```python
from build123d import *

# Parameters (mm, degrees)
BOSS_EXTRUDE1_DEPTH       = 38
BOSS_EXTRUDE1_2_DEPTH     = 38
SKETCH2_W                 = 42.2
SKETCH2_H                 = 5.9
BOSS_EXTRUDE2_DEPTH       = 2
BOSS_EXTRUDE3_DEPTH       = 18
SKETCH4_W                 = 42.2
SKETCH4_H                 = 40
BOSS_EXTRUDE4_DEPTH       = 2
SKETCH5_W                 = 38.2
SKETCH5_H                 = 11.95
CUT_EXTRUDE1_DEPTH        = 81.281509747
SKETCH6_W                 = 2
SKETCH6_H                 = 10
BOSS_EXTRUDE5_DEPTH       = 2
SKETCH7_W                 = 2
SKETCH7_H                 = 10
BOSS_EXTRUDE6_DEPTH       = 2
SKETCH8_W                 = 10
SKETCH8_H                 = 2
BOSS_EXTRUDE7_DEPTH       = 2
SKETCH9_W                 = 10
SKETCH9_H                 = 2
BOSS_EXTRUDE8_DEPTH       = 38
M3X0_5_TAPPED_HOLE1_D     = 2.5
M3X0_5_TAPPED_HOLE1_DEPTH = 7.9
M3X0_5_TAPPED_HOLE2_D     = 2.5
M3X0_5_TAPPED_HOLE2_DEPTH = 7.9


with BuildPart() as part:
    # Sketch1 → Boss-Extrude1 (new body)
    with BuildSketch(Plane(origin=(0, 0, 0), x_dir=(1, 0, 0), z_dir=(0, 1, 0))):
        Polygon((-62.898983402, -26.09346473), (-62.898983402, -24.19346473), (-60.898983402, -24.19346473), (-60.898983402, -22.19346473), (-64.898983402, -22.19346473), (-64.898983402, -28.09346473), (-60.898983402, -28.09346473), (-60.898983402, -26.09346473), align=None)
    extrude(amount=BOSS_EXTRUDE1_DEPTH)



with BuildPart() as body_2:
    # Sketch1 → Boss-Extrude1 2 (new body)
    with BuildSketch(Plane(origin=(0, 0, 0), x_dir=(1, 0, 0), z_dir=(0, 1, 0))):
        Polygon((-26.698983402, -22.19346473), (-26.698983402, -24.19346473), (-24.698983402, -24.19346473), (-24.698983402, -26.09346473), (-26.698983402, -26.09346473), (-26.698983402, -28.09346473), (-22.698983402, -28.09346473), (-22.698983402, -22.19346473), align=None)
    extrude(amount=BOSS_EXTRUDE1_2_DEPTH)


with BuildPart() as part_1:
    add(part.part)

    add(body_2.part)  # Boss-Extrude2 merges body 2
    # Sketch2 → Boss-Extrude2 (add)
    with BuildSketch(Plane(origin=(0, 0, 0), x_dir=(1, 0, 0), z_dir=(0, 1, 0))):
        with Locations((-43.798983402, -25.14346473)):
            Rectangle(SKETCH2_W, SKETCH2_H)
    extrude(amount=-BOSS_EXTRUDE2_DEPTH)

    # Sketch3 → Boss-Extrude3 (add)
    with BuildSketch(Plane(origin=(0, 0, 22.19346473), x_dir=(-1, 0, 0), z_dir=(0, 0, -1))):
        Polygon((24.698983402, 38), (22.698983402, 38), (22.698983402, -2), (64.898983402, -2), (64.898983402, 38), (62.898983402, 38), (62.898983402, 0), (24.698983402, 0), align=None)
    extrude(amount=BOSS_EXTRUDE3_DEPTH)

    # Sketch4 → Boss-Extrude4 (add)
    with BuildSketch(Plane(origin=(0, 0, 4.19346473), x_dir=(-1, 0, 0), z_dir=(0, 0, -1))):
        with Locations((43.798983402, 18)):
            Rectangle(SKETCH4_W, SKETCH4_H)
    extrude(amount=BOSS_EXTRUDE4_DEPTH)

    # Sketch5 → Cut-Extrude1 (cut, through all)
    with BuildSketch(Plane(origin=(0, 0, 0), x_dir=(1, 0, 0), z_dir=(0, 1, 0))):
        with Locations((-43.798983402, -10.16846473)):
            Rectangle(SKETCH5_W, SKETCH5_H)
    extrude(amount=-CUT_EXTRUDE1_DEPTH, mode=Mode.SUBTRACT)

    # Sketch6 → Boss-Extrude5 (add)
    with BuildSketch(Plane(origin=(-60.898983402, 0, 0), x_dir=(0, 0, -1), z_dir=(1, 0, 0))):
        with Locations((-27.09346473, 24)):
            Rectangle(SKETCH6_W, SKETCH6_H)
        with Locations((-23.19346473, 24)):
            Rectangle(SKETCH6_W, SKETCH6_H)
        with Locations((-27.09346473, 14)):
            Rectangle(SKETCH6_W, SKETCH6_H)
        with Locations((-23.19346473, 14)):
            Rectangle(SKETCH6_W, SKETCH6_H)
    extrude(amount=BOSS_EXTRUDE5_DEPTH)

    # Sketch7 → Boss-Extrude6 (add)
    with BuildSketch(Plane.ZY.offset(26.698983402)):
        with Locations((27.09346473, 24)):
            Rectangle(SKETCH7_W, SKETCH7_H)
        with Locations((27.09346473, 14)):
            Rectangle(SKETCH7_W, SKETCH7_H)
        with Locations((23.19346473, 14)):
            Rectangle(SKETCH7_W, SKETCH7_H)
        with Locations((23.19346473, 24)):
            Rectangle(SKETCH7_W, SKETCH7_H)
    extrude(amount=BOSS_EXTRUDE6_DEPTH)

    # Sketch8 → Boss-Extrude7 (add)
    with BuildSketch(Plane(origin=(0, 0, 0), x_dir=(1, 0, 0), z_dir=(0, 1, 0))):
        with Locations((-48.798983402, -23.19346473)):
            Rectangle(SKETCH8_W, SKETCH8_H)
        with Locations((-38.798983402, -23.19346473)):
            Rectangle(SKETCH8_W, SKETCH8_H)
        with Locations((-48.798983402, -27.09346473)):
            Rectangle(SKETCH8_W, SKETCH8_H)
        with Locations((-38.798983402, -27.09346473)):
            Rectangle(SKETCH8_W, SKETCH8_H)
    extrude(amount=BOSS_EXTRUDE7_DEPTH)

    # Sketch9 → Boss-Extrude8 (add)
    with BuildSketch(Plane(origin=(0, 0, 0), x_dir=(1, 0, 0), z_dir=(0, 1, 0))):
        with Locations((-57.898983402, -21.19346473)):
            Rectangle(SKETCH9_W, SKETCH9_H)
        with Locations((-29.698983402, -21.19346473)):
            Rectangle(SKETCH9_W, SKETCH9_H)
    extrude(amount=BOSS_EXTRUDE8_DEPTH)

    # M3x0.5 Tapped Hole1
    with Locations(Plane(origin=(-57.898983402, 33, 20.19346473), x_dir=(-1, 0, 0), z_dir=(0, 0, -1))):
        with Locations((0, 0), (0, -28)):
            Hole(M3X0_5_TAPPED_HOLE1_D / 2, depth=M3X0_5_TAPPED_HOLE1_DEPTH)

    # M3x0.5 Tapped Hole2
    with Locations(Plane(origin=(-29.698983402, 33, 20.19346473), x_dir=(-1, 0, 0), z_dir=(0, 0, -1))):
        with Locations((0, 0), (0, -28)):
            Hole(M3X0_5_TAPPED_HOLE2_D / 2, depth=M3X0_5_TAPPED_HOLE2_DEPTH)


solid = part_1.part
```
Design review of the part built by this model. Coordinates are the model's own, in mm. A direction names the side the tool comes from. Give positions to 0.01 mm unless a question says otherwise; leave off trailing zeros. Loops run counter-clockwise (first coordinate to the right, second up) from the corner with the lowest first, then second, coordinate; pieces in that order, holes last. Notation, with made-up numbers: (62, -38) -> (109, -38) arc R23 cw to (109, 0) -> close; hole circle Ø9 at (-40, 17). An arc over 180 degrees is marked (long way). Write each question's results on one line, items separated by ' | '.
Q1. Take a section at C-C, the plane x = -43. Write out the cut boundary in (y, z).
Reply:
outline: (-2, 2.19) -> (38, 2.19) -> (38, 4.19) -> (-2, 4.19) -> close; (-2, 16.14) -> (0, 16.14) -> (0, 22.19) -> (2, 22.19) -> (2, 24.19) -> (0, 24.19) -> (0, 26.09) -> (2, 26.09) -> (2, 28.09) -> (-2, 28.09) -> close
Q2. The part is to be moulded in two halves that separate along Z. For faces 1 (the face through (-26, 19, 24.193)), 2 (the face through (-26.699, 33, 23)), 3 (the face through (-44, 18, 2.193)), say which applies: +Z half, -Z half, draft (parallel to the pull), parting line (faces both ways), or undercut.
Reply:
face 1: undercut | face 2: draft | face 3: -Z half
Q3. Take a section at B-B, the plane y = 1. Give the number of separate pieces and of enclosed holes in the cut face, plus the area to 3 significant figures.
Reply:
separate pieces: 2 | enclosed holes: 1 | area: 316 mm²
Q4. For pin 1 Ø1.8 at (x, z) = (-38, 24.5) entering from +Y; pin 2 Ø1.5 at (x, z) = (-30, 13.5) entering from -Y; pin 3 Ø2.5 at (x, y) = (-32, 16) entering from +Z; pin 4 Ø1 at (x, z) = (-60, 27) entering from +Y, all flat-tipped, find the tip position at first contact; note any pin that passes through.
Reply:
pin 1: stops at y = 2 | pin 2: passes through | pin 3: stops at z = 22.19 | pin 4: stops at y = 29
Q5. Wall thickness on L1, parallel to Z at x = -27.5, y = 10.5; L2, parallel to X at y = 28, z = 18.5; L3, parallel to X at y = 13, z = 24: over which ranges is each line inside the solid? List them lowest first.
Reply:
L1: z = 2.19 to 4.19, 20.19 to 24.19, 26.09 to 28.09 | L2: x = -64.9 to -62.9, -24.7 to -22.7 | L3: x = -64.9 to -58.9, -28.7 to -22.7
Q6. Machinability: for faces 4 (the face through (-33.799, 1, 23)), 5 (the face through (-44, -1, 16.143)), 6 (the face through (-60.899, 4, 23)), which of the approach directions +Z, -Z, +X, -X, +Y, -Y give a long, thin tool a straight path to every point of the face, cutting with its end or side? Answer none if there is none.
Reply:
face 4: +Z, +Y | face 5: +Y, -Y | face 6: +Z
Q7. Take a section at A-A, the plane z = 6.75. Write out the cut boundary in (x, y).
Reply:
outline: (-64.9, -2) -> (-62.9, -2) -> (-62.9, 38) -> (-64.9, 38) -> close; (-24.7, -2) -> (-22.7, -2) -> (-22.7, 38) -> (-24.7, 38) -> close
